```python
from build123d import *

# Parameters (mm, degrees)
SKETCH1_R           = 110
BOSS_EXTRUDE1_DEPTH = 20
CUT_EXTRUDE2_DEPTH  = 20
SKETCH2_R           = 10.1
CUT_EXTRUDE3_DEPTH  = 20
FILLET1_R           = 10
SCALE1_SCALE        = 0.5


with BuildPart() as part:
    # Sketch1 → Boss-Extrude1 (new body)
    with BuildSketch(Plane(origin=(0, 0, 0), x_dir=(0, 0, -1), z_dir=(1, 0, 0))):
        Circle(SKETCH1_R)
    extrude(amount=BOSS_EXTRUDE1_DEPTH)

    # Sketch3 → Cut-Extrude2 (cut)
    with BuildSketch(Plane(origin=(0, 0, 0), x_dir=(0, 0, -1), z_dir=(1, 0, 0))):
        with BuildLine():
            Line((113.492219185, -10), (30, -10))
            ThreePointArc((30, -10), (20, 0), (30, 10))
            Line((30, 10), (113.492219185, 10))
            ThreePointArc((113.492219185, 10), (123.492219185, 0), (113.492219185, -10))
        make_face()
    extrude(amount=CUT_EXTRUDE2_DEPTH, mode=Mode.SUBTRACT)

    # Sketch2 → Cut-Extrude3 (cut)
    with BuildSketch(Plane(origin=(0, 0, 0), x_dir=(0, 0, -1), z_dir=(1, 0, 0))):
        Circle(SKETCH2_R)
    extrude(amount=CUT_EXTRUDE3_DEPTH, mode=Mode.SUBTRACT)

    # Fillet1
    fillet1_edges = [part.edges().sort_by_distance(p)[0] for p in [
        (20, 0, 110),
        (0, 0, 110),
    ]]
    fillet(fillet1_edges, radius=FILLET1_R - 0.0001)  # a hair under: the kernel refuses the full size


with BuildPart() as part_1:
    # Scale1: scaled about (0, 0, 0)
    add(part.part.scale(SCALE1_SCALE))


solid = part_1.part
```
Geometry: final body of the model. Coordinates: model frame, mm. A direction names the side the tool comes from. Round coordinates to 2 decimals unless told otherwise and drop trailing zeros. Loops run counter-clockwise (first coordinate to the right, second up) from the corner with the lowest first, then second, coordinate; pieces in that order, holes last. Notation, with made-up numbers: (67.25, 33.25) -> (104.25, 33.25) arc R9 ccw to (104.25, 39.25) -> close; hole circle Ø10 at (45.25, 6.25). An arc over 180 degrees is marked (long way). Write each question's results on one line, items separated by ' | '.
Item 1: Pull-direction query (Z, two-part tool) for faces 1 (the face through (5, 5, -35)), 2 (the face through (5, 0, -10)), 3 (the face through (4.93, 1.517, -4.817)); classes: pulls with the +Z half, pulls with the -Z half, needs draft (parallel to the pull), parting line crosses it, or undercut.
Answers below:
face 1: needs draft | face 2: pulls with the -Z half | face 3: undercut
Item 2: Line query: probe 1 along Y at (x, z) = (5.25, 0); probe 2 along Y at (x, z) = (5.25, -41); probe 3 along X at (y, z) = (-48.5, 14). Output: solid intervals per line, ascending. Write a range as [from, to].
Answers below:
probe 1: y = [-54.99, -5.05], [5.05, 54.99] | probe 2: y = [-36.65, -5], [5, 36.65] | probe 3: x = [0.02, 9.98]
Item 3: Set-up query: faces 4 (the face through (10, -10, 1)), 5 (the face through (5, -5, -35)). Return all of +Z, -Z, +X, -X, +Y, -Y with unobstructed straight access to the full face (end or side cutting, diameter ignored); none if empty.
Answers below:
face 4: +Z, -Z, +X, +Y, -Y | face 5: -Z, +X, -X
Item 4: Cut plane C-C on x = 7. Return the cut outline in (y, z).
Answers below:
outline: (-5, -54.35) -> (-5, -15) arc R5 cw to (5, -15) -> (5, -54.35) arc R54.58 ccw (long way) to start; hole circle Ø10.1 at (0, 0)
Item 5: Pin query (flat end, axial travel): pin 1 Ø6 at (x, y) = (3.5, 41.5) entering from +Z; pin 2 Ø3 at (x, z) = (3, 19) entering from -Y; pin 3 Ø2 at (x, z) = (2, -30) entering from -Y. Return the tip coordinate at first contact, or that it passes through.
Answers below:
pin 1: stops at z = 39.11 | pin 2: stops at y = -51.91 | pin 3: stops at y = -45.89
